Drawing for the job (mm, zero at the part's lowest x, y, z). A direction names the side the tool comes from. Round coordinates to 2 decimals unless told otherwise and drop trailing zeros. Loops run counter-clockwise (first coordinate to the right, second up) from the corner with the lowest first, then second, coordinate; pieces in that order, holes last. Notation, with made-up numbers: M 36,74.25 L 65,74.25 A38 cw 65,112.25 Z; hole C 55,25 d1. An arc over 180 degrees is marked long. Use a Markdown table: item, result. Add a question column.
Q1. Mould opens along X. For the marked faces 3, 4, 5 and 6 say: +X half, -X half, draft (parallel to the pull), parting line (faces both ways), or undercut.
Q2. Cut at B-B (y = 2.5). Give the cut face in (x, z), plus the area to 3 significant figures.
Q3. Cut at A-A (z = 8.5). Give the cut face in (x, y).
Q4. Pin check, flat tips, straight feed: pin 1 (3 mm diameter, centred on x = 8, y = 3, fed in from -Z); pin 2 (3 mm diameter, centred on x = 16.5, y = 3.5, fed in from +Z). Stop position of each tip, or through.
Q5. Cut at D-D (y = 6). Give the cut face in (x, z).
Q6. Cut at C-C (z = 4.5). Give the cut face in (x, y).
Q7. Tool access for the marked faces 1 and 2: list every direction of +Z, -Z, +X, -X, +Y, -Y with a clear straight run to the whole face (end or side of a thin tool).
Q8. Probe line 1 (X direction, y = 3.75, z = 4.25); line 2 (Z direction, x = 16, y = 0.75); line 3 (Z direction, x = 2, y = 0.75). List the from-to ranges inside material, lowest first. Write a range as from..to.
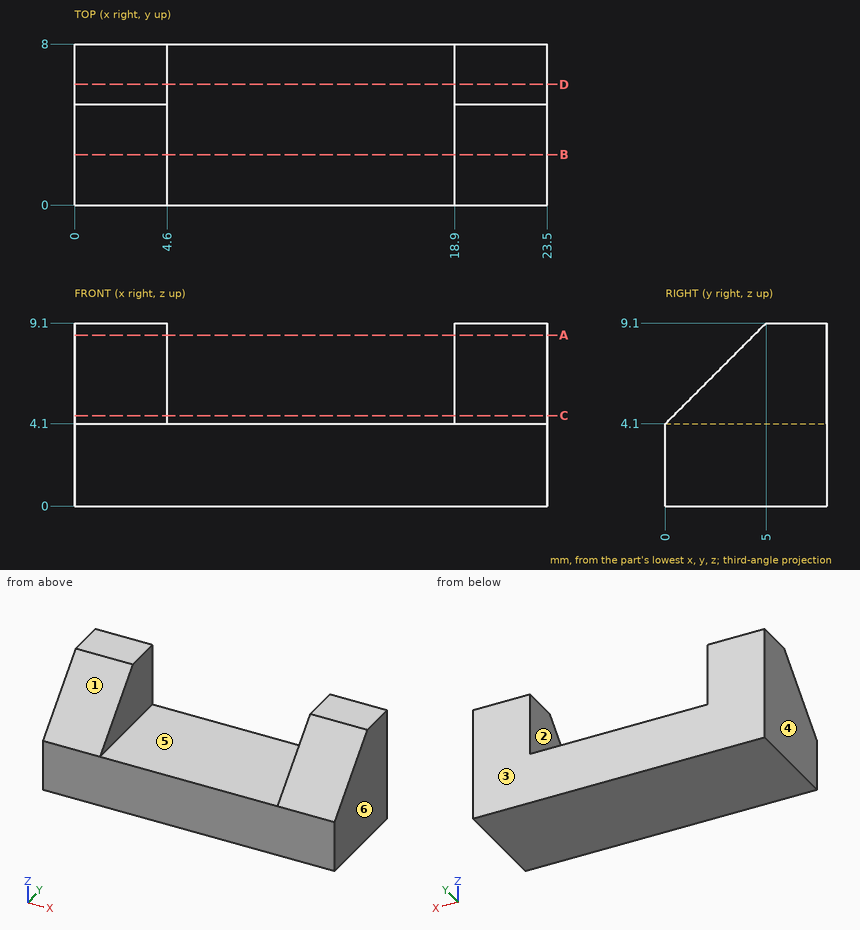
Checked values:
| question | item | result |
|---|---|---|
| 1 | face 3 | draft |
| 1 | face 4 | -X half |
| 1 | face 5 | undercut |
| 1 | face 6 | +X half |
| 2 | outline | M 0,0 L 23.5,0 L 23.5,6.6 L 18.9,6.6 L 18.9,4.1 L 4.6,4.1 L 4.6,6.6 L 0,6.6 Z |
| 2 | area | 119 mm^2 |
| 3 | outline | M 0,4.4 L 4.6,4.4 L 4.6,8 L 0,8 Z; M 18.9,4.4 L 23.5,4.4 L 23.5,8 L 18.9,8 Z |
| 4 | pin 1 | stops at z = 0 |
| 4 | pin 2 | stops at z = 4.1 |
| 5 | outline | M 0,0 L 23.5,0 L 23.5,9.1 L 18.9,9.1 L 18.9,4.1 L 4.6,4.1 L 4.6,9.1 L 0,9.1 Z |
| 6 | outline | M 0,0.4 L 4.6,0.4 L 4.6,8 L 0,8 Z; M 18.9,0.4 L 23.5,0.4 L 23.5,8 L 18.9,8 Z |
| 7 | face 1 | +Z, +X, -X, -Y |
| 7 | face 2 | +Z, +Y, -Y |
| 8 | line 1 | x = 0..4.6, 18.9..23.5 |
| 8 | line 2 | z = 0..4.1 |
| 8 | line 3 | z = 0..4.85 |
